Autodesk Inventor part; units mm, degrees
ref_plane "YZ Plane" through (0, 0, 0) normal (1, 0, 0) x (0, 1, 0)
ref_plane "XZ Plane" through (0, 0, 0) normal (0, 1, 0) x (-1, 0, 0)
sketch "Sketch1" plane through (0, 0, 0) normal (0, 0, 1) x (1, 0, 0)
  line L0 (0, 0) -> (-88.9, 0)
  line L1 (-153.7877, 0) -> (0, 0)
  line L2 (-88.9, 0) -> (-88.9, -21.8948)
  line L3 (-88.9, -21.8948) -> (0, -21.8948)
  line L4 (0, -21.8948) -> (0, 0)
  dimension "d0" = 88.9
  dimension "d1" = 21.8948
revolve "Revolution1" add sketch "Sketch1" angle 360 about axis through (0, -21.8948, 0) along (0, 1, 0)
ref_plane "Work Plane1" through (0, -10.9474, -88.9) normal (0, 0, 1) x (1, 0, 0)
sketch "Sketch2" plane through (0, -10.9474, -88.9) normal (0, 0, 1) x (1, 0, 0)
  line L0 (0, 10.9474) -> (0, 0)
  dimension "d3" = 10.9474
hole "Hole1" at (0, -10.9474, -88.9) direction (0, 0, 1) diameter 4.9784 depth 12.7 tip angle 118
pattern_circular "Circular Pattern1" count 6 over 360 about axis through (0, -10, 0) along (0, 1, 0) of "Hole1"
sketch "Sketch3" plane through (0, 0, 0) normal (0, 1, 0) x (1, 0, 0)
  circle A0 centre (0, 0) radius 9.525
  point P0 (0, 0)
  dimension "d14" = 19.05
extrude "Extrusion1" cut sketch "Sketch3" against normal blind 74.6125
properties part number "Avi Bay phenolic" material "Phenolic Resin"
Check sheet for the modelled part. Datum: model origin and axes. Units: mm. A direction names the side the tool comes from. Coordinates: 2 decimals unless noted, no trailing zeros. Order: outer loops, then holes, each group sorted by start corner. A loop starts at its lowest first (then second) coordinate and runs counter-clockwise, first axis right, second up. Notation, with made-up numbers: (78, 20.25) -> (85, 20.25) arc R7 cw to (85, 31.25) -> close; hole circle Ø9 at (-20, 18.25). An arc over 180 degrees is marked (long way). Write item = value, one per line. Start each with the question number.
1) Cross-section at A-A (z = 0). Enter the section's corners in (x, y) (3 decimals).
2) Access from +Z, -Z, +X, -X, +Y, -Y to the whole of each face (thin tool, end or side, straight path). Record for faces 5 (the cylindrical face through (-7.559, -10.794, 5.796)), 6 (the cylindrical face through (0.748, -8.573, 82.461)), 7 (the conical face through (-65, -10.55, -37.34)).
3) Mould release check, pull along Z, two halves, no side actions. Record for faces 1 (the cylindrical face through (-0.748, -8.573, -82.461)), 2 (the conical face through (0.263, -11.29, 74.964)), 3 (the conical face through (64.986, -10.535, -37.37)), 4 (the conical face through (65, -10.55, 37.34)): +Z half, -Z half, draft (parallel to the pull), parting line (faces both ways), or undercut.
4) Cross-section at B-B (y = -15.5). Enter the section's corners in (x, z) (3 decimals), then the cut area to 3 significant figures.
5) Go/stop test with flat-tipped pins: P1, Ø2, axis at x = 60, z = -63.5, coming from the +Y side; P2, Ø2, axis at x = -9.5, y = -14, coming from the -Z side; P3, Ø5, axis at x = 27.5, y = -15, coming from the -Z side; P4, Ø11.5, axis at x = 0, z = 0, coming from the -Y side. Record where each tip stops, or that it passes through.
6) Cross-section at C-C (x = -48). Enter the section's corners in (y, z).
7) Cross-section at D-D (z = -32). Enter the section's corners in (x, y).
8) Material ranges on L1, parallel to Z at x = 0, y = -4.5 (3 decimals); L2, parallel to Z at x = 76, y = -9; L3, parallel to Y at x = 0, z = -83, recorded low to high.
Ans:
q1.outline = (-88.9, -21.895) -> (-9.525, -21.895) -> (-9.525, 0) -> (-88.9, 0) -> close; (9.525, -21.895) -> (88.9, -21.895) -> (88.9, 0) -> (9.525, 0) -> close
q2.face_5 = +Y, -Y
q2.face_6 = +Z
q2.face_7 = none
q3.face_1 = draft
q3.face_2 = +Z half
q3.face_3 = undercut
q3.face_4 = undercut
q4.outline = circle Ø177.8 at (0, 0); hole circle Ø19.05 at (0, 0)
q4.area = 24,500 mm²
q5.P1 = 0
q5.P2 = -88.49
q5.P3 = -85.31
q5.P4 = through
q6.outline = (-21.89, -74.83) -> (0, -74.83) -> (0, 74.83) -> (-21.89, 74.83) -> close
q7.outline = (-82.94, -21.89) -> (82.94, -21.89) -> (82.94, 0) -> (-82.94, 0) -> close
q8.L1 = -88.9 to -9.525, 9.525 to 88.9
q8.L2 = -46.12 to -45.67, -42.09 to 42.09, 45.67 to 46.12
q8.L3 = -21.89 to -13.44, -8.46 to 0
